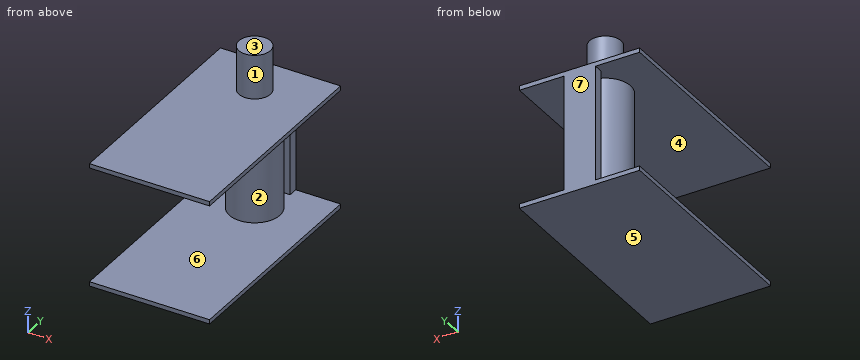
Autodesk Inventor part; units mm, degrees
ref_plane "YZ Plane" through (0, 0, 0) normal (1, 0, 0) x (0, 1, 0)
ref_plane "XZ Plane" through (0, 0, 0) normal (0, 1, 0) x (-1, 0, 0)
ref_plane "XY Plane" through (0, 0, 0) normal (0, 0, 1) x (1, 0, 0)
sketch "Sketch1" plane through (0, 0, 0) normal (0, 0, 1) x (1, 0, 0)
  line L0 (0, 0) -> (242.2769, 0)
  line L1 (242.2769, 0) -> (242.2769, 441.325)
  line L2 (242.2769, 441.325) -> (0, 441.325)
  line L3 (0, 441.325) -> (0, 0)
  dimension "d0" = 242.2769
  dimension "d1" = 441.325
extrude "Extrusion1" add sketch "Sketch1" along normal blind 8.7605
sketch "Sketch2" plane through (0, 0, 8.7605) normal (0, 0, 1) x (1, 0, 0)
  line L0 (242.2769, 441.325) -> (0, 441.325)
  line L1 (0, 441.325) -> (88.9, 441.325)
  line L2 (88.9, 441.325) -> (88.9, 422.3233)
  line L3 (88.9, 422.3233) -> (151.8437, 422.3233)
  line L4 (151.8437, 422.3233) -> (151.8437, 441.325)
  dimension "d4" = 88.9
  dimension "d5" = 19.0017
  dimension "d6" = 62.9437
extrude "Extrusion2" add sketch "Sketch2" along normal blind 231.7166
sketch "Sketch3" plane through (0, 0, 240.477) normal (0, 0, 1) x (1, 0, 0)
  line L0 (88.9, 441.325) -> (88.9, 422.3233)
  line L1 (88.9, 422.3233) -> (151.8437, 422.3233)
  line L2 (151.8437, 422.3233) -> (151.8437, 441.325)
  line L3 (151.8437, 441.325) -> (88.9, 441.325)
  line L4 (88.9, 441.325) -> (0, 441.325)
  line L5 (151.8437, 441.325) -> (151.8437, 422.3233)
  line L6 (151.8437, 422.3233) -> (88.9, 422.3233)
  line L7 (88.9, 422.3233) -> (88.9, 441.325)
  line L8 (88.9, 441.325) -> (0, 441.325)
  line L9 (0, 441.325) -> (0, 0)
  line L10 (0, 0) -> (242.2769, 0)
  line L11 (242.2769, 0) -> (242.2769, 441.325)
  line L12 (242.2769, 441.325) -> (151.8437, 441.325)
extrude "Extrusion3" add sketch "Sketch3" along normal blind 8.7605
sketch "Sketch6" plane through (0, 0, 8.7605) normal (0, 0, 1) x (1, 0, 0)
  circle A0 centre (120.3719, 355.4324) radius 50.8
extrude "Extrusion4" add sketch "Sketch6" along normal blind 231.7166
sketch "Sketch7" plane through (0, 0, 249.2375) normal (0, 0, 1) x (1, 0, 0)
  circle A0 centre (120.3719, 355.4324) radius 50.8
  circle A1 centre (120.3719, 355.4324) radius 31.75
  dimension "d15" = 63.5
extrude "Extrusion5" add sketch "Sketch7" along normal blind 88.9 contours A1
properties part number "Robotics ball launcher motor frame"
Part model, mm, in its own coordinate system. Face numbers are marked on the shaded views. A direction names the side the tool comes from. Give positions to 0.01 mm unless a question says otherwise; leave off trailing zeros. Loops run counter-clockwise (first coordinate to the right, second up) from the corner with the lowest first, then second, coordinate; pieces in that order, holes last. Notation, with made-up numbers: M 54.5,-23 L 76.5,-23 A32 ccw 76.5,6 Z; hole C -37,68 d3. An arc over 180 degrees is marked long. Put each result on its own line as item: value. Start each with the question number.
1) 3-axis set-ups, long thin cutter, end or side, ignore diameter. For the marked faces 1, 2 and 3: which of +Z, -Z, +X, -X, +Y, -Y reach the whole face in a straight line?
2) Probe probe 1 along Z at (x, y) = (187.5, 295.5); probe 2 along Y at (x, z) = (117, 206.5) (3 decimals); probe 3 along Y at (x, z) = (104, 183) (3 decimals). List the from-to ranges inside material, lowest first.
3) Saw through at A-A (x = 26). List the corners of the cut face in (y, z) (1 decimal).
4) Pull direction Z, two halves, no side cores. Call the marked faces 4, 5, 6 and 7: +Z half, -Z half, draft (parallel to the pull), parting line (faces both ways), or undercut.
5) Saw through at C-C (z = 79.5). List the corners of the cut face in (x, y) (3 decimals).
6) Saw through at B-B (y = 199). List the corners of the cut face in (x, z), then the cut area to 3 significant figures.
7) Flat gauge pins, fed straight in: pin 1 (15 mm diameter, centred on y = 429, z = 139.5, fed in from +X); pin 2 (5 mm diameter, centred on x = 191, y = 89.5, fed in from +Z); pin 3 (19 mm diameter, centred on x = 106.5, z = 134, fed in from -Y). Where does each tip first touch, or does it go through?
8) Saw through at D-D (y = 376). List the corners of the cut face in (x, z), then the cut area to 3 significant figures.
Numbers:
1. face 1: +Z
1. face 2: none
1. face 3: +Z, +X, -X, +Y, -Y
2. probe 1: 0 to 8.76, 240.48 to 249.24
2. probe 2: 304.744 to 406.12, 422.323 to 441.325
2. probe 3: 307.343 to 403.522, 422.323 to 441.325
3. outline: M 0,0 L 441.3,0 L 441.3,8.8 L 0,8.8 Z; M 0,240.5 L 441.3,240.5 L 441.3,249.2 L 0,249.2 Z
4. face 4: undercut
4. face 5: -Z half
4. face 6: undercut
4. face 7: draft
5. outline: C 120.372,355.432 d101.6; M 88.9,422.323 L 151.844,422.323 L 151.844,441.325 L 88.9,441.325 Z
6. outline: M 0,0 L 242.28,0 L 242.28,8.76 L 0,8.76 Z; M 0,240.48 L 242.28,240.48 L 242.28,249.24 L 0,249.24 Z
6. area: 4,240 mm^2
7. pin 1: x = 151.84
7. pin 2: z = 249.24
7. pin 3: y = 304.82
8. outline: M 0,0 L 242.28,0 L 242.28,8.76 L 166.82,8.76 L 166.82,240.48 L 242.28,240.48 L 242.28,249.24 L 144.56,249.24 L 144.56,338.14 L 96.18,338.14 L 96.18,249.24 L 0,249.24 L 0,240.48 L 73.92,240.48 L 73.92,8.76 L 0,8.76 Z
8. area: 30,100 mm^2
